from build123d import *

# Parameters (mm, degrees)
SKETCH1_R           = 3.175
BOSS_EXTRUDE1_DEPTH = 3
SKETCH2_W           = 20
SKETCH2_H           = 3
BOSS_EXTRUDE2_DEPTH = 8
SKETCH3_W           = 3
SKETCH3_H           = 10
BOSS_EXTRUDE3_DEPTH = 8
BOSS_EXTRUDE4_DEPTH = 3
BOSS_EXTRUDE5_DEPTH = 8
FILLET1_START       = 9.218775709
FILLET1_DEPTH       = 8.281224391
FILLET1_START_2     = -10
FILLET1_2_DEPTH     = 6
FILLET2_R           = 2.5
SKETCH6_R           = 2.5
CUT_EXTRUDE1_DEPTH  = 10


with BuildPart() as part:
    # Sketch1 → Boss-Extrude1 (new body)
    with BuildSketch(Plane.XY):
        with BuildLine():
            Line((-60.325, -31.75), (-60.325, -44.45))
            Line((-60.325, -44.45), (-48.025, -44.45))
            Line((-48.025, -44.45), (-21.676299295, -24.294954915))
            ThreePointArc((-21.676299295, -24.294954915), (-9.525, -20.180354672), (2.626299295, -24.294954915))
            Line((2.626299295, -24.294954915), (28.975, -44.45))
            Line((28.975, -44.45), (41.275, -44.45))
            Line((41.275, -44.45), (41.275, -31.75))
            ThreePointArc((41.275, -31.75), (36.515027492, -27.39513634), (32.512762317, -22.33509195))
            ThreePointArc((32.512762317, -22.33509195), (30.830682399, -16.998296592), (32.278938689, -11.593360767))
            ThreePointArc((32.278938689, -11.593360767), (35.521007508, 0), (32.278938689, 11.593360767))
            ThreePointArc((32.278938689, 11.593360767), (30.830682399, 16.998296592), (32.512762317, 22.33509195))
            ThreePointArc((32.512762317, 22.33509195), (36.515027492, 27.39513634), (41.275, 31.75))
            Line((41.275, 31.75), (41.275, 44.45))
            Line((41.275, 44.45), (28.975, 44.45))
            Line((28.975, 44.45), (2.626299295, 24.294954915))
            ThreePointArc((2.626299295, 24.294954915), (-9.525, 20.180354672), (-21.676299295, 24.294954915))
            Line((-21.676299295, 24.294954915), (-48.025, 44.45))
            Line((-48.025, 44.45), (-60.325, 44.45))
            Line((-60.325, 44.45), (-60.325, 31.75))
            ThreePointArc((-60.325, 31.75), (-48.881491961, 17.673557002), (-44.789364565, 0))
            ThreePointArc((-44.789364565, 0), (-48.881491961, -17.673557002), (-60.325, -31.75))
        make_face()
        with Locations((-53.975, -38.1)):
            Circle(SKETCH1_R, mode=Mode.SUBTRACT)
        with Locations((34.925, -38.1)):
            Circle(SKETCH1_R, mode=Mode.SUBTRACT)
        with Locations((-53.975, 38.1)):
            Circle(SKETCH1_R, mode=Mode.SUBTRACT)
        with BuildLine():
            Line((-18.525, -12), (-30.525, -12))
            Line((-30.525, -12), (-30.525, 12))
            Line((-30.525, 12), (-18.525, 12))
            ThreePointArc((-18.525, 12), (-9.525, 15), (-0.525, 12))
            Line((-0.525, 12), (29.475, 12))
            Line((29.475, 12), (29.475, -12))
            Line((29.475, -12), (-0.525, -12))
            ThreePointArc((-0.525, -12), (-9.525, -15), (-18.525, -12))
        make_face(mode=Mode.SUBTRACT)
        with Locations((34.925, 38.1)):
            Circle(SKETCH1_R, mode=Mode.SUBTRACT)
    extrude(amount=BOSS_EXTRUDE1_DEPTH)

    # Sketch2 → Boss-Extrude2 (add)
    with BuildSketch(Plane.YZ.offset(20.475)):
        with BuildLine():
            Line((10, 17.5), (10, 14.5))
            add(Edge.make_bspline(
                [(10, 14.5), (16.044635902, 14.437929649), (14.184736767, 5.689745318), (18.589920917, 3)],
                knots=[0, 0, 0, 0, 1, 1, 1, 1], degree=3))
            Line((18.589920917, 3), (24.346709493, 3))
            Line((24.346709493, 3), (20.153292557, 5.560443148))
            add(Edge.make_bspline(
                [(10.030804376, 17.499841844), (10.580284275, 17.494199418), (11.690825904, 17.381169352), (13.744868646, 16.699236551), (15.740064205, 15.05007217), (17.01264364, 12.797944804), (17.78675167, 10.651473672), (18.380074772, 8.685818255), (18.969741662, 7.060430969), (19.488563299, 6.172247499), (19.869226233, 5.760648886), (20.051080137, 5.622852657), (20.153292557, 5.560443148)],
                knots=[0, 0, 0, 0, 0.0625, 0.125, 0.25, 0.375, 0.5, 0.625, 0.75, 0.875, 0.9375, 1, 1, 1, 1], degree=3))
            Line((10.030804376, 17.499841844), (10, 17.5))
        make_face()
        with Locations((0, 16)):
            Rectangle(SKETCH2_W, SKETCH2_H)
        with BuildLine():
            add(Edge.make_bspline(
                [(-10, 14.5), (-16.044635902, 14.437929649), (-14.184736767, 5.689745318), (-18.589920917, 3)],
                knots=[0, 0, 0, 0, 1, 1, 1, 1], degree=3))
            Line((-10, 14.5), (-10, 17.5))
            Line((-10, 17.5), (-10.030804376, 17.499841844))
            add(Edge.make_bspline(
                [(-10.030804376, 17.499841844), (-10.580284275, 17.494199418), (-11.690825904, 17.381169352), (-13.744868646, 16.699236551), (-15.740064205, 15.05007217), (-17.01264364, 12.797944804), (-17.78675167, 10.651473672), (-18.380074772, 8.685818255), (-18.969741662, 7.060430969), (-19.488563299, 6.172247499), (-19.869226233, 5.760648886), (-20.051080137, 5.622852657), (-20.153292557, 5.560443148)],
                knots=[0, 0, 0, 0, 0.0625, 0.125, 0.25, 0.375, 0.5, 0.625, 0.75, 0.875, 0.9375, 1, 1, 1, 1], degree=3))
            Line((-20.153292557, 5.560443148), (-24.346709493, 3))
            Line((-24.346709493, 3), (-18.589920917, 3))
        make_face()
    extrude(amount=BOSS_EXTRUDE2_DEPTH)

    # Sketch3 → Boss-Extrude3 (add)
    with BuildSketch(Plane.ZY.offset(19.525)):
        with Locations((16, 5)):
            Rectangle(SKETCH3_W, SKETCH3_H)
        with Locations((16, -5)):
            Rectangle(SKETCH3_W, SKETCH3_H)
        with BuildLine():
            add(Edge.make_bspline(
                [(14.5, 10), (14.31563917, 16.035707977), (5.493486467, 14.05293238), (3, 18.609732698)],
                knots=[0, 0, 0, 0, 1, 1, 1, 1], degree=3))
            Line((14.5, 10), (17.5, 10))
            Line((17.5, 10), (17.491030171, 10.04523587))
            add(Edge.make_bspline(
                [(17.491030171, 10.04523587), (17.485387745, 10.594715769), (17.372357679, 11.705257398), (16.690424877, 13.75930014), (15.041260496, 15.754495699), (12.789133131, 17.027075134), (10.642661999, 17.801183164), (8.677006582, 18.394506266), (7.051619296, 18.984173156), (6.163435825, 19.502994793), (5.751837213, 19.883657727), (5.614040983, 20.065511631), (5.551631475, 20.167724051)],
                knots=[0, 0, 0, 0, 0.0625, 0.125, 0.25, 0.375, 0.5, 0.625, 0.75, 0.875, 0.9375, 1, 1, 1, 1], degree=3))
            Line((5.551631475, 20.167724051), (3, 22.905906895))
            Line((3, 22.905906895), (3, 18.609732698))
        make_face()
    extrude(amount=BOSS_EXTRUDE3_DEPTH)

    # Sketch4 → Boss-Extrude4 (add)
    with BuildSketch(Plane(origin=(0, 0, 14.5), x_dir=(-1, 0, 0), z_dir=(0, 0, -1))):
        with BuildLine():
            Line((27.525, -18), (27.525, -10))
            Line((27.525, -10), (19.525, -10))
            ThreePointArc((19.525, -10), (21.868145751, -15.656854249), (27.525, -18))
        make_face()
    extrude(amount=-BOSS_EXTRUDE4_DEPTH)

    # Sketch5 → Boss-Extrude5 (add)
    with BuildSketch(Plane.XZ.offset(10)):
        with BuildLine():
            Line((-37.647488181, 5.560601304), (-40.424026667, 3.033030687))
            Line((-40.424026667, 3.033030687), (-36.12785247, 3.033030687))
            add(Edge.make_bspline(
                [(-27.525, 14.5), (-33.57036544, 14.381422519), (-31.574084791, 5.518855921), (-36.12785247, 3.033030687)],
                knots=[0, 0, 0, 0, 1, 1, 1, 1], degree=3))
            Line((-27.525, 14.5), (-27.525, 17.5))
            add(Edge.make_bspline(
                [(-27.525, 17.5), (-28.074479899, 17.494357574), (-29.185021529, 17.381327508), (-31.23906427, 16.699394706), (-33.234259829, 15.050230325), (-34.506839264, 12.79810296), (-35.280947294, 10.651631828), (-35.874270396, 8.685976411), (-36.463937286, 7.060589125), (-36.982758923, 6.172405654), (-37.363421857, 5.760807042), (-37.545275761, 5.623010812), (-37.647488181, 5.560601304)],
                knots=[0, 0, 0, 0, 0.0625, 0.125, 0.25, 0.375, 0.5, 0.625, 0.75, 0.875, 0.9375, 1, 1, 1, 1], degree=3))
        make_face()
    extrude(amount=BOSS_EXTRUDE5_DEPTH)

    # Fillet1: read off the stored shape, not the designer's step
    # Fillet1 outline → Fillet1 (add)
    with BuildSketch(Plane.XY.offset(FILLET1_START)):
        with BuildLine():
            Line((-27.525, -10), (-27.525, -5))
            ThreePointArc((-27.525, -5), (-28.989466094, -8.535533906), (-32.525, -10))
            Line((-32.525, -10), (-27.525, -10))
        make_face()
    extrude(amount=FILLET1_DEPTH)

    # Fillet1 2 outline → Fillet1 2 (cut)
    with BuildSketch(Plane(origin=(0, 0, 0), x_dir=(1, 0, 0), z_dir=(0, 1, 0)).offset(FILLET1_START_2)):
        with BuildLine():
            Line((-32.525, -17.5000001), (-27.525, -17.5))
            add(Edge.make_bspline(
                [(-27.525, -17.5), (-28.074479899, -17.494357574), (-29.185021529, -17.381327508), (-30.968007207, -16.789384412), (-32.004283714, -16.043301537), (-32.525, -15.550477548)],
                knots=[0, 0, 0, 0, 0.0625, 0.125, 0.217009321, 0.217009321, 0.217009321, 0.217009321], degree=3))
            Line((-32.525, -15.550477548), (-32.525, -17.5000001))
        make_face()
        with BuildLine():
            Line((-27.525, -9.218775709), (-32.525000028, -9.218775718))
            add(Edge.make_bspline(
                [(-32.525000028, -9.218775718), (-31.668443392, -11.933356908), (-30.719340028, -14.437344269), (-27.525, -14.5)],
                knots=[0.47160514, 0.47160514, 0.47160514, 0.47160514, 1, 1, 1, 1], degree=3))
            Line((-27.525, -14.5), (-27.525, -9.218775709))
        make_face()
    extrude(amount=FILLET1_2_DEPTH, mode=Mode.SUBTRACT)

    # Fillet2
    fillet2_edges = [part.edges().sort_by_distance(p)[0] for p in [
        (-18.525, 12, 1.5),
        (-30.525, 12, 1.5),
        (-30.525, -12, 1.5),
        (-18.525, -12, 1.5),
        (-0.525, -12, 1.5),
        (29.475, -12, 1.5),
        (29.475, 12, 1.5),
        (-0.525, 12, 1.5),
    ]]
    fillet(fillet2_edges, radius=FILLET2_R)

    # Sketch6 → Cut-Extrude1 (cut)
    with BuildSketch(Plane(origin=(0, 0, 14.5), x_dir=(-1, 0, 0), z_dir=(0, 0, -1))):
        with Locations(Location((24.525, -5.5, 0), (0, 0, 90))):
            Circle(SKETCH6_R)
        with Locations(Location((24.525, 5.5, 0), (0, 0, 90))):
            Circle(SKETCH6_R)
        with Locations(Location((-25.475, -5.5, 0), (0, 0, 90))):
            Circle(SKETCH6_R)
        with Locations(Location((-25.475, 5.5, 0), (0, 0, 90))):
            Circle(SKETCH6_R)
    extrude(amount=-CUT_EXTRUDE1_DEPTH, mode=Mode.SUBTRACT)


solid = part.part
Check sheet for the modelled part. Datum: model origin and axes. Units: mm. A direction names the side the tool comes from. Give positions to 0.01 mm unless a question says otherwise; leave off trailing zeros. Write each loop counter-clockwise with the first axis right and the second up, starting at its lowest first coordinate (ties: lowest second). Pieces come first, ordered by that corner, then holes. Notation, with made-up numbers: (-25.5, 43.5) -> (25.5, 43.5) arc R25 ccw to (25.5, 72.5) -> close; hole circle Ø1 at (64, -2.5). An arc over 180 degrees is marked (long way). Use one line per item in the form item = value. Start each with the question number.
1. Section check A-A (x = -10). Record the cut outline in (y, z), and give its area (3 significant figures).
2. Section check C-C (y = 5.5). Record the cut outline in (x, z) (3 decimals), and give its area (3 significant figures).
3. Access from +Z, -Z, +X, -X, +Y, -Y to the whole of each face (thin tool, end or side, straight path). Record for faces 4 (the flat face through (-23.47, 21.52, 4.29)), 5 (the cylindrical face through (28.72, 11.29, 1.52)), 6 (the flat face through (-34, -18, 11)), 7 (the cylindrical face through (-29.77, 11.29, 1.52)), 8 (the cylindrical face through (-21.806, -15.594, 15.979)).
4. Mould release check, pull along X, two halves, no side actions. Record for faces 1 (the flat face through (-39.02, -13.94, 4.31)), 2 (the flat face through (-19.525, 8, 15)), 3 (the cylindrical face through (36.577, -27.461, 1.479)): pulls with the +X half, pulls with the -X half, needs draft (parallel to the pull), parting line crosses it, or undercut.
5. Thickness scan on line 1 along X through (y, z) = (-5.5, 16.2) (3 decimals); line 2 along Z through (x, y) = (-37.5, 32.5); line 3 along Y through (x, z) = (25, 3.5). Record the ranges inside material, lowest first. Write a range as from..to.
6. Section check B-B (y = 29.5). Record the cut outline in (x, z), and give its area (3 significant figures).
7. Go/stop test with flat-tipped pins: P1, Ø6.5, axis at x = -24.5, y = -6.5, coming from the -Z side; P2, Ø1.5, axis at y = 22, z = 3.5, coming from the +X side; P3, Ø10, axis at x = 34.925, y = -38.1, coming from the +Z side. Record where each tip stops, or that it passes through.
Conclusion:
q1.outline = (-20.19, 0) -> (-14.99, 0) -> (-14.99, 3) -> (-20.19, 3) -> close; (14.99, 0) -> (20.19, 0) -> (20.19, 3) -> (14.99, 3) -> close
q1.area = 31.2 mm²
q2.outline = (-45.167, 0) -> (-30.525, 0) -> (-30.525, 3) -> (-45.167, 3) -> close; (-27.525, 14.5) -> (-27.025, 14.5) -> (-27.025, 17.5) -> (-27.525, 17.5) -> close; (-22.025, 14.5) -> (-19.525, 14.5) -> (-19.525, 17.5) -> (-22.025, 17.5) -> close; (20.475, 14.5) -> (22.975, 14.5) -> (22.975, 17.5) -> (20.475, 17.5) -> close; (27.975, 14.5) -> (28.475, 14.5) -> (28.475, 17.5) -> (27.975, 17.5) -> close; (29.475, 0) -> (34.834, 0) -> (34.834, 3) -> (29.475, 3) -> close
q2.area = 78.0 mm²
q3.face_4 = +Z, -X, +Y
q3.face_5 = -Z
q3.face_6 = +Z, -X, -Y
q3.face_7 = +Z, -Z
q3.face_8 = +Z, -Y
q4.face_1 = pulls with the -X half
q4.face_2 = undercut
q4.face_3 = pulls with the +X half
q5.line_1 = -27.55..-27.025, -22.025..-19.525, 20.475..22.975, 27.975..28.475
q5.line_2 = 0..3
q5.line_3 = -23.53..-17.91, 17.91..23.53
q6.outline = (-57.67, 0) -> (-28.48, 0) -> (-28.48, 3) -> (-57.67, 3) -> close; (9.43, 0) -> (38.62, 0) -> (38.62, 3) -> (9.43, 3) -> close
q6.area = 175 mm²
q7.P1 = 14.49
q7.P2 = 32.66
q7.P3 = 3
